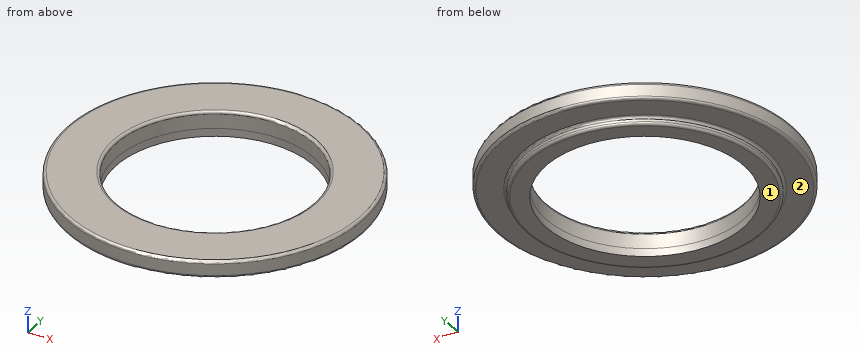
```python
from build123d import *

# Parameters (mm, degrees)
F0_R     = 56
F0_R_2   = 37.5
F1_DEPTH = 6.5
F2_R     = 45
F2_R_2   = 37.5
F3_DEPTH = 3
F4_R     = 1


with BuildPart() as f1:
    # F0 (on Top) → F1 (new body)
    with BuildSketch(Plane.XY):
        Circle(F0_R)
        Circle(F0_R_2, mode=Mode.SUBTRACT)
    extrude(amount=F1_DEPTH)

    # F2 (on Top) → F3 (join)
    with BuildSketch(Plane.XY):
        Circle(F2_R)
        Circle(F2_R_2, mode=Mode.SUBTRACT)
    extrude(amount=-F3_DEPTH)

    # F4
    f4_edges = [f1.edges().sort_by_distance(p)[0] for p in [
        (-56, 0, 6.5),
        (-45, 0, -3),
        (-45, 0, 0),
        (-37.5, 0, 6.5),
        (-56, 0, 0),
    ]]
    fillet(f4_edges, radius=F4_R)


solid = f1.part
```
Part model, mm, in its own coordinate system. Face numbers are marked on the shaded views. A direction names the side the tool comes from. Give positions to 0.01 mm unless a question says otherwise; leave off trailing zeros. Loops run counter-clockwise (first coordinate to the right, second up) from the corner with the lowest first, then second, coordinate; pieces in that order, holes last. Notation, with made-up numbers: M -32,-32 L 0,-32 A24 ccw 0,-12 Z; hole C 88,44.25 d4. An arc over 180 degrees is marked long. Return JSON: item names as keys, results as strings.
1) 3-axis set-ups, long thin cutter, end or side, ignore diameter. For the marked faces 1 and 2: which of +Z, -Z, +X, -X, +Y, -Y reach the whole face in a straight line?
Calculated:
{"face 1": "-Z, +X, -X, +Y, -Y", "face 2": "-Z"}
2) Flat gauge pins, fed straight in: pin 1 Ø3 at (y, z) = (-14, -1) entering from +X; pin 2 Ø1 at (y, z) = (-19.5, 0.5) entering from +X; pin 3 Ø2 at (y, z) = (20.5, 4) entering from +X. Where does each tip first touch, or does it go through?
Calculated:
{"pin 1": "stops at x = 54.15", "pin 2": "stops at x = 52.62", "pin 3": "stops at x = 52.5"}
3) Saw through at A-A, the plane x = 0. List the corners of the cut face in (y, z), then the cut area to 3 significant figures.
Calculated:
{"outline": "M -56,1 A1 ccw -55,0 L -46,0 A1 cw -45,-1 L -45,-2 A1 ccw -44,-3 L -37.5,-3 L -37.5,5.5 A1 ccw -38.5,6.5 L -55,6.5 A1 ccw -56,5.5 Z; M 37.5,-3 L 44,-3 A1 ccw 45,-2 L 45,-1 A1 cw 46,0 L 55,0 A1 ccw 56,1 L 56,5.5 A1 ccw 55,6.5 L 38.5,6.5 A1 ccw 37.5,5.5 Z", "area": "284 mm2"}
4) Drill centre lines: line 1 (Y direction, x = 0, z = -1.95); line 2 (Y direction, x = 0, z = 2); line 3 (Z direction, x = 5.5, y = 50). Where is each one in solid material? Low to high.
Calculated:
{"line 1": "y = -45 to -37.5, 37.5 to 45", "line 2": "y = -56 to -37.5, 37.5 to 56", "line 3": "z = 0 to 6.5"}
5) Saw through at C-C, the plane z = 3.25. List the corners of the cut face in (x, y), then the cut area to 3 significant figures.
Calculated:
{"outline": "C 0,0 d112; hole C 0,0 d75", "area": "5,430 mm2"}
